from build123d import *

# Parameters (mm, degrees)
BOSS_EXTRUDE1_DEPTH                             = 6.35
CSK_FOR_M4_FLAT_HEAD_MACHINE_SCREW1_D           = 4.3
CSK_FOR_M4_FLAT_HEAD_MACHINE_SCREW1_CSINK_D     = 9.4
CSK_FOR_M4_FLAT_HEAD_MACHINE_SCREW1_CSINK_ANGLE = 90
CHAMFER1_SIZE                                   = 16
SKETCH6_W                                       = 10
SKETCH6_H                                       = 6
BOSS_EXTRUDE2_DEPTH                             = 6.35
FILLET5_R                                       = 8
M3X0_5_TAPPED_HOLE1_D                           = 2.5
FILLET6_START                                   = -1
FILLET6_DEPTH                                   = 8
SKETCH18_W                                      = 25
SKETCH18_H                                      = 19
BOSS_EXTRUDE4_DEPTH                             = 6.35
FILLET12_R                                      = 3
M3X0_5_TAPPED_HOLE2_D                           = 2.5
FILLET13_R                                      = 50
FILLET14_R                                      = 16


with BuildPart() as part:
    # Sketch1 → Boss-Extrude1 (new body)
    with BuildSketch(Plane(origin=(0, 0, 0), x_dir=(1, 0, 0), z_dir=(0, 1, 0))):
        Polygon((-5, 171.5), (5, 171.5), (5, 152.5), (152.5, 152.5), (152.5, -168.5), (142.5, -168.5), (142.5, -152.5), (-142.5, -152.5), (-142.5, -168.5), (-152.5, -168.5), (-152.5, 152.5), (-5, 152.5), align=None)
    extrude(amount=BOSS_EXTRUDE1_DEPTH)

    # CSK for M4 Flat Head Machine Screw1 (through all)
    with Locations(Plane(origin=(0, 6.35, 0), x_dir=(1, 0, 0), z_dir=(0, 1, 0))):
        with Locations((0, 166.5), (-147.5, -163.5), (147.5, -163.5)):
            CounterSinkHole(CSK_FOR_M4_FLAT_HEAD_MACHINE_SCREW1_D / 2, CSK_FOR_M4_FLAT_HEAD_MACHINE_SCREW1_CSINK_D / 2, counter_sink_angle=CSK_FOR_M4_FLAT_HEAD_MACHINE_SCREW1_CSINK_ANGLE)

    # Chamfer1
    chamfer1_edges = [part.edges().sort_by_distance(p)[0] for p in [
        (142.5, 3.175, 152.5),
        (-142.5, 3.175, 152.5),
    ]]
    chamfer(chamfer1_edges, length=CHAMFER1_SIZE - 0.0001)  # a hair under: the kernel refuses the full size

    # Sketch6 → Boss-Extrude2 (add)
    with BuildSketch(Plane(origin=(0, 6.35, 0), x_dir=(1, 0, 0), z_dir=(0, 1, 0))):
        with Locations((-147.5, 155.5)):
            Rectangle(SKETCH6_W, SKETCH6_H)
        with Locations((147.5, 155.5)):
            Rectangle(SKETCH6_W, SKETCH6_H)
    extrude(amount=-BOSS_EXTRUDE2_DEPTH)

    # Fillet5
    # the kernel refuses this fillet: 8 mm, written as the material it adds along each edge
    with BuildSketch(Plane(origin=(142.5, 6.35, -152.5), x_dir=(0, 0, -1), z_dir=(0, -1, 0))) as fillet5_piece_1:
        with BuildLine():
            CenterArc((8, -7.745966692), FILLET5_R, 104.477512186, 75.522487814)
            Line((0, -7.745966692), (-0.16, -7.745966692))
            Line((-0.16, -7.745966692), (-0.16, 0))
            Line((-0.16, 0), (0, 0.16))
            ThreePointArc((0, 0.16), (3, 0.16), (5.96, 0.154919334))
            Line((5.96, 0.154919334), (6, 0))
        make_face()
    extrude(amount=6.35)
    with BuildSketch(Plane(origin=(-142.5, 6.35, -152.5), x_dir=(1, 0, 0), z_dir=(0, -1, 0))) as fillet5_piece_2:
        with BuildLine():
            CenterArc((7.745966692, -8), FILLET5_R, 90, 75.522487814)
            Line((0, -6), (-0.154919334, -5.96))
            ThreePointArc((-0.154919334, -5.96), (-0.16, -3), (-0.16, 0))
            Line((-0.16, 0), (0, 0.16))
            Line((0, 0.16), (7.745966692, 0.16))
            Line((7.745966692, 0.16), (7.745966692, 0))
        make_face()
    extrude(amount=6.35)

    # M3x0.5 Tapped Hole1 (through all)
    with Locations(Plane(origin=(0, 6.35, 0), x_dir=(1, 0, 0), z_dir=(0, 1, 0))):
        with Locations((-147.5, 154), (147.5, 154), (137.107695155, -157.5), (-137.107695155, -157.5), (0, 155.5)):
            Hole(M3X0_5_TAPPED_HOLE1_D / 2)

    # Fillet6: read off the stored shape, not the designer's step
    # Fillet6 outline → Fillet6 (cut)
    with BuildSketch(Plane(origin=(0, 0, 0), x_dir=(1, 0, 0), z_dir=(0, 1, 0)).offset(FILLET6_START)):
        with BuildLine():
            ThreePointArc((152.5, -163.5), (151.035533906, -167.035533906), (147.5, -168.5))
            Line((147.5, -168.5), (152.5, -168.5))
            Line((152.5, -168.5), (152.5, -163.5))
        make_face()
        with BuildLine():
            ThreePointArc((144.571067812, -168.5), (142.65765065, -168.119397663), (141.035533906, -167.035533906))
            Line((141.035533906, -167.035533906), (142.5, -168.5))
            Line((142.5, -168.5), (144.571067812, -168.5))
        make_face()
        with BuildLine():
            ThreePointArc((-141.035533906, -167.035533906), (-142.65765065, -168.119397663), (-144.571067812, -168.5))
            Line((-144.571067812, -168.5), (-142.5, -168.5))
            Line((-142.5, -168.5), (-141.035533906, -167.035533906))
        make_face()
        with BuildLine():
            Line((-152.5, -168.5), (-147.5, -168.5))
            ThreePointArc((-147.5, -168.5), (-151.035533906, -167.035533906), (-152.5, -163.5))
            Line((-152.5, -163.5), (-152.5, -168.5))
        make_face()
    extrude(amount=FILLET6_DEPTH, mode=Mode.SUBTRACT)

    # Sketch18 → Boss-Extrude4 (add)
    with BuildSketch(Plane.XZ):
        with Locations((17.5, -162)):
            Rectangle(SKETCH18_W, SKETCH18_H)
        with Locations((-17.5, -162)):
            Rectangle(SKETCH18_W, SKETCH18_H)
    extrude(amount=-BOSS_EXTRUDE4_DEPTH)

    # Fillet12
    fillet12_edges = [part.edges().sort_by_distance(p)[0] for p in [
        (30, 3.175, -171.5),
        (-30, 3.175, -171.5),
        (-142.5, 3.175, -158.5),
        (-152.5, 3.175, -158.5),
        (142.5, 3.175, -158.5),
        (152.5, 3.175, -158.5),
    ]]
    fillet(fillet12_edges, radius=FILLET12_R)

    # M3x0.5 Tapped Hole2 (through all)
    with Locations(Plane(origin=(0, 6.35, 0), x_dir=(1, 0, 0), z_dir=(0, 1, 0))):
        with Locations((27, 154.5), (-27, 168.5), (-27, 158.5)):
            Hole(M3X0_5_TAPPED_HOLE2_D / 2)

    # Fillet13
    # the kernel refuses this fillet: 50 mm, written as the material it adds along each edge
    with BuildSketch(Plane(origin=(126.5001, 0, 152.5), x_dir=(-1, 0, 0), z_dir=(0, 1, 0))) as fillet13_piece_1:
        with BuildLine():
            CenterArc((20.710446515, 50), FILLET13_R, 225.146645298, 44.853354702)
            Line((-14.554286856, 14.554286856), (-15.259581524, 13.845372594))
            Line((-15.259581524, 13.845372594), (-0.707106781, -0.707106781))
            Line((-0.707106781, -0.707106781), (0, -1))
            Line((0, -1), (20.710446515, -1))
            Line((20.710446515, -1), (20.710446515, 0))
        make_face()
    extrude(amount=6.35)
    with BuildSketch(Plane(origin=(-126.5001, 0, 152.5), x_dir=(-0.7071067811865476, 0, 0.7071067811865476), z_dir=(0, 1, 0))) as fillet13_piece_2:
        with BuildLine():
            CenterArc((20.710841887, 49.999836231), FILLET13_R, 225, 44.853354702)
            Line((-14.644497172, 14.644497172), (-15.351603953, 13.937390391))
            Line((-15.351603953, 13.937390391), (-0.707106781, -0.707106781))
            Line((-0.707106781, -0.707106781), (0, -1))
            Line((0, -1), (20.580310423, -0.999996725))
            Line((20.580310423, -0.999996725), (20.582869863, 0))
        make_face()
    extrude(amount=6.35)

    # Fillet14
    fillet14_edges = [part.edges().sort_by_distance(p)[0] for p in [
        (30, 3.175, -152.5),
        (-30, 3.175, -152.5),
    ]]
    fillet(fillet14_edges, radius=FILLET14_R - 0.0001)  # a hair under: the kernel refuses the full size


solid = part.part
Geometry: final body of the model. Coordinates: model frame, mm. A direction names the side the tool comes from. Round coordinates to 2 decimals unless told otherwise and drop trailing zeros. Loops run counter-clockwise (first coordinate to the right, second up) from the corner with the lowest first, then second, coordinate; pieces in that order, holes last.
Q1. Section A-A on y = 1.75. State how many separate pieces and enclosed holes the cut face has, plus the area to 3 significant figures.
Q2. Section C-C on x = -115. Return loops of the section in (y, z), plus the area to 3 significant figures.
Q3. Material intervals for L1, parallel to Z at x = -147.5, y = 1.5; L2, parallel to Z at x = -27, y = 3.75; L3, parallel to X at y = 2.9, z = 163.5, sorted ascending.
Q4. Pull-direction query (X, two-part tool) for faces 1 (the flat face through (0, 6.35, 9)), 2 (the cylindrical face through (125.118, 3.131, 156.387)); classes: released by +X, released by -X, zero draft, split by the parting line, or undercut.
Q5. Pin query (flat end, axial travel): P1, Ø5.5, axis at x = 147.5, z = 163.5, coming from the +Y side; P2, Ø4, axis at x = -137.11, z = 157.5, coming from the -Y side; P3, Ø2.5, axis at x = -146, y = 4, coming from the -Z side; P4, Ø2, axis at x = -98.5, y = 1, coming from the +Z side. Return the tip coordinate at first contact, or that it passes through.
Q6. Section B-B on x = 98. Return loops of the section in (y, z), plus the area to 3 significant figures.
Q7. Access query for faces 3 (the conical face through (149.3, 3.92, 164.88)), 4 (the cylindrical face through (-124.611, 3.131, 156.178)), 5 (the cylindrical face through (-34.563, 3.219, -157.311)). Directions: +Z, -Z, +X, -X, +Y, -Y. A direction counts if a zero-diameter tool reaches every point of the face in a straight line with its end or side. Return the directions, or none.
Evaluation:
1. separate pieces: 1
1. enclosed holes: 11
1. area: 95,000 mm2
2. outline: (0, -152.5) - (6.35, -152.5) - (6.35, 153.36) - (0, 153.36) - close
2. area: 1,940 mm2
3. L1: z = -158.5 to -155.25, -152.75 to 161.35, 165.65 to 168.5
3. L2: z = -171.5 to -169.75, -167.25 to -159.75, -157.25 to 152.5
3. L3: x = -152.5 to -149.65, -145.35 to -137.08, 137.08 to 145.35, 149.65 to 152.5
4. face 1: zero draft
4. face 2: undercut
5. P1: stops at y = 4.4
5. P2: stops at y = 0
5. P3: stops at z = -158.5
5. P4: stops at z = 152.5
6. outline: (0, -152.5) - (6.35, -152.5) - (6.35, 152.5) - (0, 152.5) - close
6. area: 1,940 mm2
7. face 3: +Y
7. face 4: +Z, +Y, -Y
7. face 5: -Z, +Y, -Y
